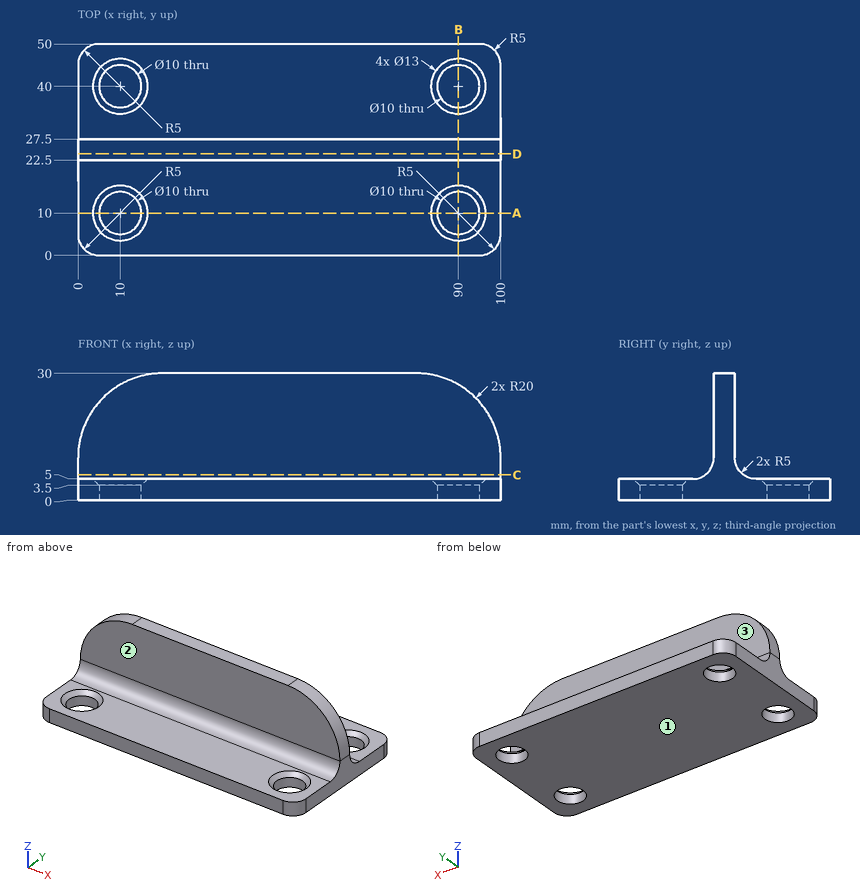
The drawing under review shows one solid part. Ordinate dimensions are in mm from its lowest x, y, z. A direction names the side the tool comes from. Coordinates: 2 decimals unless noted, no trailing zeros. Write each loop counter-clockwise with the first axis right and the second up, starting at its lowest first coordinate (ties: lowest second). Pieces come first, ordered by that corner, then holes. Notation, with made-up numbers: M -5.75,44 L 51.25,44 A25 ccw 51.25,73 Z; hole C 41.25,-24.75 d2. An arc over 180 degrees is marked long. Put each result on its own line as item: value.
1) Add section C-C on z = 6. Give the boundary of the cut face in (x, y), then the cut area to 3 significant figures.
Computed:
outline: M 0,20.5 L 100,20.5 L 100,29.5 L 0,29.5 Z
area: 900 mm2
2) Add section B-B on x = 90. Give the boundary of the cut face in (y, z).
Computed:
outline: M 0,0 L 5,0 L 5,3.5 L 3.5,5 L 0,5 Z; M 15,0 L 35,0 L 35,3.5 L 33.5,5 L 32.5,5 A5 cw 27.5,10 L 27.5,27.32 L 22.5,27.32 L 22.5,10 A5 cw 17.5,5 L 16.5,5 L 15,3.5 Z; M 45,0 L 50,0 L 50,5 L 46.5,5 L 45,3.5 Z
3) Add section D-D on y = 24. Give the boundary of the cut face in (x, z).
Computed:
outline: M 0,0 L 100,0 L 100,10 A20 ccw 80,30 L 20,30 A20 ccw 0,10 Z
4) Add section A-A on y = 10. Give the boundary of the cut face in (x, z).
Computed:
outline: M 0,0 L 5,0 L 5,3.5 L 3.5,5 L 0,5 Z; M 15,0 L 85,0 L 85,3.5 L 83.5,5 L 16.5,5 L 15,3.5 Z; M 95,0 L 100,0 L 100,5 L 96.5,5 L 95,3.5 Z
5) Wall thickness on probe 1 along Y at (x, z) = (10, 1.65); probe 2 along X at (y, z) = (43.5, 4); probe 3 along Z at (x, y) = (71.5, 11.5): over which ranges is each line inside the solid? List them lowest first. Write a range as [from, to].
Computed:
probe 1: y = [0, 5], [15, 35], [45, 50]
probe 2: x = [0, 5.76], [14.24, 85.76], [94.24, 100]
probe 3: z = [0, 5]
6) For the marked faces 1, 2 and 3, list the 3-axis set-ups (+Z, -Z, +X, -X, +Y, -Y) from which the entire face can be reached by the end or side of a thin tool; tool diameter is ignored.
Computed:
face 1: -Z, +X, -X, +Y, -Y
face 2: +Z, +X, -X, -Y
face 3: +Z, +X, -X, +Y
7) Clearance check with flat-ended pins moving along their axes: pin 1 Ø3 at (x, y) = (16, 26) entering from +Z; pin 2 Ø2 at (x, z) = (71, 24.5) entering from +Y; pin 3 Ø6 at (x, z) = (61, 17) entering from -Y. State where each tip first meets the part, or that it passes through.
Computed:
pin 1: stops at z = 29.84
pin 2: stops at y = 27.5
pin 3: stops at y = 22.5
